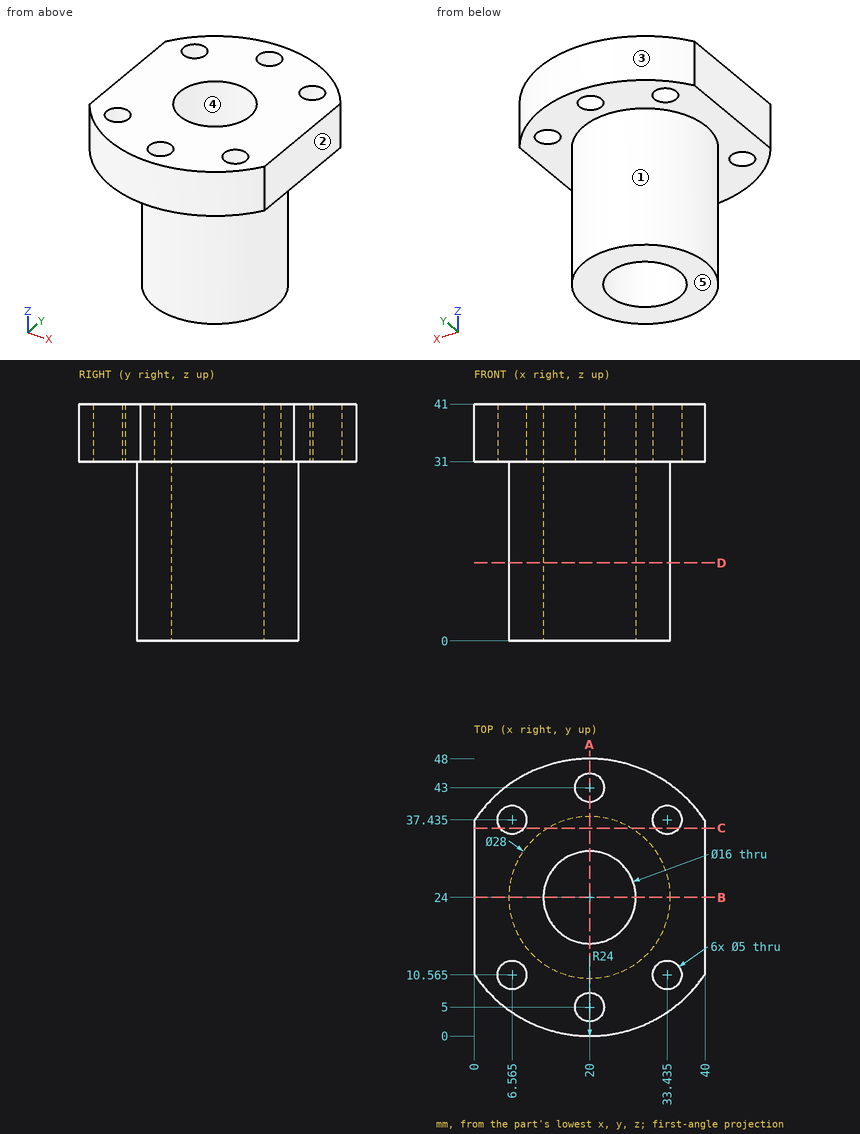
Source: three-view drawing plus pictorial views. Frame: mm from the lowest corner of the part. A direction names the side the tool comes from. Coordinates: 2 decimals unless noted, no trailing zeros. Order: outer loops, then holes, each group sorted by start corner. A loop starts at its lowest first (then second) coordinate and runs counter-clockwise, first axis right, second up. Notation, with made-up numbers: M 71,87.25 L 113,87.25 A12 cw 113,100.25 Z; hole C -3.75,-20 d7. An arc over 180 degrees is marked long. One line per question, with ' | ' between items.
Item 1: Section C-C (y = 36). Output: boundary loops of the cut face in (x, z), then the cut area to 3 significant figures.
Geometry results:
outline: M 0,31 L 4.52,31 L 4.52,41 L 0,41 Z; M 8.61,31 L 12.79,31 L 12.79,0 L 27.21,0 L 27.21,31 L 31.39,31 L 31.39,41 L 8.61,41 Z; M 35.48,31 L 40,31 L 40,41 L 35.48,41 Z | area: 765 mm^2
Item 2: Ray query, line 1 along Y through (x, z) = (20, 25); line 2 along Y through (x, z) = (21, 16.5); line 3 along Z through (x, y) = (6, 23). Return the intervals inside material, ascending.
Geometry results:
line 1: y = 10 to 16, 32 to 38 | line 2: y = 10.04 to 16.06, 31.94 to 37.96 | line 3: z = 31 to 41
Item 3: Reachability of the marked faces 1 and 2 from +Z, -Z, +X, -X, +Y, -Y: full face, straight path, thin tool, end or side. Return the list, or none.
Geometry results:
face 1: -Z | face 2: +Z, -Z, +X, +Y, -Y
Item 4: Section D-D (z = 13.5). Output: boundary loops of the cut face in (x, y).
Geometry results:
outline: C 20,24 d28; hole C 20,24 d16
Item 5: Pin query (flat end, axial travel): pin 1 (6 mm diameter, centred on x = 25.5, z = 26, fed in from -Y) (3 decimals); pin 2 (20 mm diameter, centred on x = 22.5, y = 26, fed in from -Z); pin 3 (3 mm diameter, centred on x = 36, y = 14, fed in from -Z); pin 4 (12 mm diameter, centred on x = 35, z = 22, fed in from -Y). Return the tip coordinate at first contact, or that it passes through.
Geometry results:
pin 1: stops at y = 10.225 | pin 2: stops at z = 0 | pin 3: stops at z = 31 | pin 4: stops at y = 13.28
Item 6: Section A-A (x = 20). Output: boundary loops of the cut face in (y, z).
Geometry results:
outline: M 0,31 L 2.5,31 L 2.5,41 L 0,41 Z; M 7.5,31 L 10,31 L 10,0 L 16,0 L 16,41 L 7.5,41 Z; M 32,0 L 38,0 L 38,31 L 40.5,31 L 40.5,41 L 32,41 Z; M 45.5,31 L 48,31 L 48,41 L 45.5,41 Z
Item 7: Section B-B (y = 24). Output: boundary loops of the cut face in (x, z).
Geometry results:
outline: M 0,31 L 6,31 L 6,0 L 12,0 L 12,41 L 0,41 Z; M 28,0 L 34,0 L 34,31 L 40,31 L 40,41 L 28,41 Z
Item 8: Draft query along Y for the marked faces 3, 4 and 5. Return one class per face: released by +Y, released by -Y, zero draft, split by the parting line, or undercut.
Geometry results:
face 3: released by +Y | face 4: undercut | face 5: zero draft
